Check sheet for the modelled part. Datum: model origin and axes. Units: mm. Face numbers are marked on the shaded views. A direction names the side the tool comes from. Give positions to 0.01 mm unless a question says otherwise; leave off trailing zeros. Loops run counter-clockwise (first coordinate to the right, second up) from the corner with the lowest first, then second, coordinate; pieces in that order, holes last. Notation, with made-up numbers: (-30.5, 45.5) - (9.5, 45.5) arc R27 cw to (9.5, 76.5) - close; hole circle Ø7 at (0.25, 53.5). An arc over 180 degrees is marked (long way). Answer in a Markdown table with one row per item. Add a question column.
(1) Sectioned sample at D-D on y = -6.75. Enter the section's corners in (x, z) (3 decimals).
(2) Sectioned sample at C-C on z = 3.5. Enter the section's corners in (x, y) (3 decimals).
(3) Sectioned sample at B-B on x = -3.75. Enter the section's corners in (y, z).
(4) Thickness scan on L1, parallel to Y at x = -3.25, z = -13.25; L2, parallel to Z at x = 0, y = 0.65 (3 decimals); L3, parallel to Y at x = 1, z = 7.75. Record the ranges inside material, lowest first.
(5) Draft check along Y on the marked faces 1, 2, 3 and 4. Enter one of: released by +Y, released by -Y, zero draft, split by the parting line, or undercut.
(6) Sectioned sample at A-A on z = -13. Enter the section's corners in (x, y) (3 decimals), then the cut area to 3 significant figures.
(7) Set-up check for the marked faces 5, 6, 7 and 8: record each of +Z, -Z, +X, -X, +Y, -Y from which the full face is reachable in a straight line by a thin tool's end or side.
(8) Go/stop test with flat-tipped pins: P1, Ø1.5, axis at x = 4, y = -10, coming from the -Z side; P2, Ø2, axis at x = -3.5, z = -9.5, coming from the +Y side; P3, Ø1.5, axis at x = 0.5, z = -5.5, coming from the +Y side. Record where each tip stops, or that it passes through.
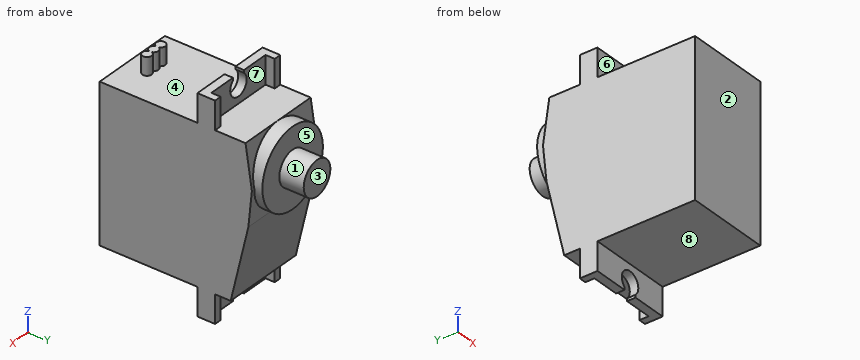
from build123d import *

# Parameters (mm, degrees)
SKETCH2_W           = 11.85
SKETCH2_H           = 21.8
BOSS_EXTRUDE1_DEPTH = 13.8
SKETCH3_W           = 11.85
SKETCH3_H           = 29.7
BOSS_EXTRUDE2_DEPTH = 1.2
SKETCH4_R           = 1.5
CUT_EXTRUDE11_DEPTH = 1.2
SKETCH5_W           = 2
SKETCH5_H           = 2
CUT_EXTRUDE12_DEPTH = 1.2
SKETCH6_R           = 5.5
BOSS_EXTRUDE3_DEPTH = 7.65
SKETCH7_R           = 2.42
BOSS_EXTRUDE4_DEPTH = 3.45
BOSS_EXTRUDE5_DEPTH = 11.85
SKETCH9_W           = 1
SKETCH9_H           = 3.95
BOSS_EXTRUDE6_DEPTH = 1.3
BOSS_EXTRUDE7_DEPTH = 2.5


with BuildPart() as part:
    # Sketch2 → Boss-Extrude1 (new body)
    with BuildSketch(Plane(origin=(0, 0, 0), x_dir=(1, 0, 0), z_dir=(0, 1, 0))):
        Rectangle(SKETCH2_W, SKETCH2_H)
    extrude(amount=-BOSS_EXTRUDE1_DEPTH)

    # Sketch3 → Boss-Extrude2 (add)
    with BuildSketch(Plane(origin=(0, 0, 0), x_dir=(1, 0, 0), z_dir=(0, 1, 0))):
        Rectangle(SKETCH3_W, SKETCH3_H)
    extrude(amount=BOSS_EXTRUDE2_DEPTH)

    # Sketch4 → Cut-Extrude11 (cut)
    with BuildSketch(Plane(origin=(0, 1.2, 0), x_dir=(1, 0, 0), z_dir=(0, 1, 0))):
        with Locations((0, 13.355)):
            Circle(SKETCH4_R)
        with Locations((0, -13.355)):
            Circle(SKETCH4_R)
    extrude(amount=-CUT_EXTRUDE11_DEPTH, mode=Mode.SUBTRACT)

    # Sketch5 → Cut-Extrude12 (cut)
    with BuildSketch(Plane(origin=(0, 1.2, 0), x_dir=(1, 0, 0), z_dir=(0, 1, 0))):
        with Locations((0, 14.85)):
            Rectangle(SKETCH5_W, SKETCH5_H)
        with Locations((0, -14.85)):
            Rectangle(SKETCH5_W, SKETCH5_H)
    extrude(amount=-CUT_EXTRUDE12_DEPTH, mode=Mode.SUBTRACT)

    # Sketch6 → Boss-Extrude3 (add)
    with BuildSketch(Plane(origin=(0, 1.2, 0), x_dir=(1, 0, 0), z_dir=(0, 1, 0))):
        with Locations((0, -5.4)):
            Circle(SKETCH6_R)
    extrude(amount=BOSS_EXTRUDE3_DEPTH)

    # Sketch7 → Boss-Extrude4 (add)
    with BuildSketch(Plane(origin=(0, 8.85, 0), x_dir=(1, 0, 0), z_dir=(0, 1, 0))):
        with Locations((0, -5.4)):
            Circle(SKETCH7_R)
    extrude(amount=BOSS_EXTRUDE4_DEPTH)

    # Sketch8 → Boss-Extrude5 (add)
    with BuildSketch(Plane(origin=(5.925, 0, 0), x_dir=(0, 0, -1), z_dir=(1, 0, 0))):
        Polygon((-10.9, 1.2), (-10.9, 6.8), (-4.9, 7.7), (0.1, 7.2), (10.9, 4.7), (10.9, 1.2), align=None)
    extrude(amount=-BOSS_EXTRUDE5_DEPTH)

    # Sketch9 → Boss-Extrude6 (add)
    with BuildSketch(Plane(origin=(0, 1.2, 0), x_dir=(1, 0, 0), z_dir=(0, 1, 0))):
        with Locations((5.425, -12.875)):
            Rectangle(SKETCH9_W, SKETCH9_H)
        with Locations((-5.425, -12.875)):
            Rectangle(SKETCH9_W, SKETCH9_H)
        with Locations((-5.425, 12.875)):
            Rectangle(SKETCH9_W, SKETCH9_H)
        with Locations((5.425, 12.875)):
            Rectangle(SKETCH9_W, SKETCH9_H)
    extrude(amount=BOSS_EXTRUDE6_DEPTH)

    # Sketch10 → Boss-Extrude7 (add)
    with BuildSketch(Plane.XY.offset(10.9)):
        with BuildLine():
            ThreePointArc((-0.625, -10.928535711), (0, -11.4), (0.625, -10.928535711))
            ThreePointArc((0.625, -10.928535711), (1.9, -10.75), (0.625, -10.571464289))
            ThreePointArc((0.625, -10.571464289), (0, -10.1), (-0.625, -10.571464289))
            ThreePointArc((-0.625, -10.571464289), (-1.9, -10.75), (-0.625, -10.928535711))
        make_face()
    extrude(amount=BOSS_EXTRUDE7_DEPTH)


solid = part.part
Reply:
| question | item | result |
|---|---|---|
| 1 | outline | (-5.925, -10.9) - (5.925, -10.9) - (5.925, 10.9) - (-5.925, 10.9) - close |
| 2 | outline | (-5.925, -13.8) - (5.925, -13.8) - (5.925, 7.56) - (5.161, 7.56) - (5.161, 8.85) - (1.499, 8.85) - (1.499, 12.3) - (-1.499, 12.3) - (-1.499, 8.85) - (-5.161, 8.85) - (-5.161, 7.56) - (-5.925, 7.56) - close |
| 3 | outline | (-13.8, -10.9) - (0, -10.9) - (0, -14.85) - (1.2, -14.85) - (1.2, -10.9) - (4.7, -10.9) - (7.2, -0.1) - (7.35, 1.38) - (8.85, 1.38) - (8.85, 9.42) - (7.02, 9.42) - (6.8, 10.9) - (1.2, 10.9) - (1.2, 14.85) - (0, 14.85) - (0, 10.9) - (-13.8, 10.9) - close |
| 4 | L1 | 0 to 1.2 |
| 4 | L2 | -11.855 to 11.855 |
| 4 | L3 | -13.8 to 8.85 |
| 5 | face 1 | zero draft |
| 5 | face 2 | released by -Y |
| 5 | face 3 | released by +Y |
| 5 | face 4 | undercut |
| 6 | outline | (-5.925, 0) - (-1.457, 0) - (-1.457, 1.2) - (-4.925, 1.2) - (-4.925, 2.5) - (-5.925, 2.5) - close; (1.457, 0) - (5.925, 0) - (5.925, 2.5) - (4.925, 2.5) - (4.925, 1.2) - (1.457, 1.2) - close |
| 6 | area | 13.3 mm^2 |
| 7 | face 5 | +Y |
| 7 | face 6 | +Z, +X, -X |
| 7 | face 7 | +Z, +Y |
| 7 | face 8 | -Z, +X, -X, -Y |
| 8 | P1 | z = -10.9 |
| 8 | P2 | y = 5.26 |
| 8 | P3 | y = 6.12 |
